```python
from build123d import *

# Parameters (mm, degrees)
CROQUIS1_R              = 25
SALIENTE_EXTRUIR1_DEPTH = 30


with BuildPart() as part:
    # Croquis1 → Saliente-Extruir1 (new body)
    with BuildSketch(Plane(origin=(0, 0, 0), x_dir=(1, 0, 0), z_dir=(0, 1, 0))):
        with BuildLine():
            Line((-65.797376832, 25.36524745), (-63.002208753, 26.454758997))
            ThreePointArc((-63.002208753, 26.454758997), (-56.557387251, 8.427488435), (-51.143577362, -9.935759386))
            Line((-51.143577362, -9.935759386), (-27.717597065, -3.966713114))
            ThreePointArc((-27.717597065, -3.966713114), (27.133039517, 6.913621813), (-26.236106677, -9.780935868))
            Line((-26.236106677, -9.780935868), (-49.662086973, -15.74998214))
            ThreePointArc((-49.662086973, -15.74998214), (-45.628225194, -34.464847013), (-42.660438023, -53.378081728))
            Line((-42.660438023, -53.378081728), (-45.636154363, -53.759017766))
            ThreePointArc((-45.636154363, -53.759017766), (-53.297041908, -13.580328562), (-65.797376832, 25.36524745))
        make_face()
        Circle(CROQUIS1_R, mode=Mode.SUBTRACT)
    extrude(amount=SALIENTE_EXTRUIR1_DEPTH)


solid = part.part
```
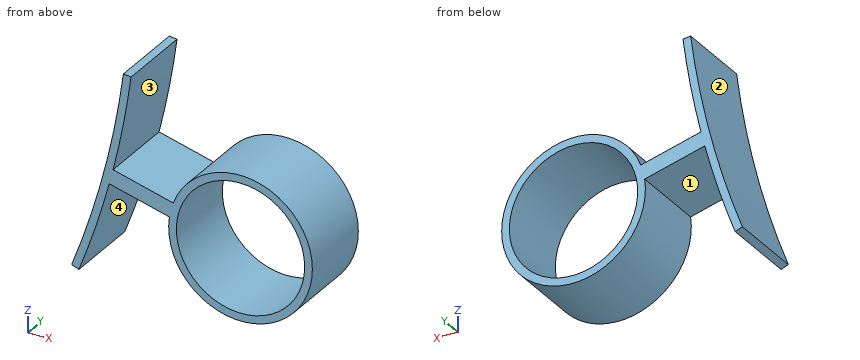
Geometry: final body of the model. Coordinates: model frame, mm. Face numbers are marked on the shaded views. A direction names the side the tool comes from. Round coordinates to 2 decimals unless told otherwise and drop trailing zeros. Order: outer loops, then holes, each group sorted by start corner. A loop starts at its lowest first (then second) coordinate and runs counter-clockwise, first axis right, second up. Notation, with made-up numbers: M 33,-1.75 L 77,-1.75 A7 cw 77,6.25 Z; hole C 59,-4.75 d11. An arc over 180 degrees is marked long. Use one line per item in the form item = value. Start each with the question number.
Q1. Mould query, pull axis X, two halves, no side actions, for the marked faces 1 and 2. Classes: +X half, -X half, draft (parallel to the pull), parting line (faces both ways), or undercut.
Q2. Cut plane C-C (y = 16.5). Return loops of the section in (x, z), and give its area (3 significant figures).
Q3. Cut plane A-A (x = 0). Return loops of the section in (y, z), and give its area (3 significant figures).
Q4. Pin query (flat end, axial travel): pin 1 Ø10 at (y, z) = (10.5, -6.5) entering from -X; pin 2 Ø5 at (y, z) = (24, 32.5) entering from +X; pin 3 Ø4 at (y, z) = (25.5, 42) entering from -X. Return the tip coordinate at first contact, or that it passes through.
Q5. Access query for the marked faces 3 and 4. Directions: +Z, -Z, +X, -X, +Y, -Y. A direction counts if a zero-diameter tool reaches every point of the face in a straight line with its end or side. Return the directions, or none.
Q6. Cut plane D-D (x = -13). Return loops of the section in (y, z).
Q7. Cut plane B-B (z = 18). Return loops of the section in (x, y), and give its area (3 significant figures).
Q8. Material intervals for line 1 (X direction, y = 19, z = 0); line 2 (X direction, y = 26.5, z = -19); line 3 (Z direction, x = 0, y = 13), sorted ascending. Write a range as [from, to].
Geometry results:
q1.face_1 = undercut
q1.face_2 = -X half
q2.outline = M -65.8,-25.37 L -63,-26.45 A338 ccw -51.14,9.94 L -27.72,3.97 A28 ccw long -26.24,9.78 L -49.66,15.75 A338 ccw -42.66,53.38 L -45.64,53.76 A335 cw Z; hole C 0,0 d50
q2.area = 891 mm^2
q3.outline = M 0,-28 L 30,-28 L 30,-25 L 0,-25 Z; M 0,25 L 30,25 L 30,28 L 0,28 Z
q3.area = 180 mm^2
q4.pin_1 = -60.74
q4.pin_2 = -45.53
q4.pin_3 = -47.69
q5.face_3 = +Y, -Y
q5.face_4 = -Z, +Y, -Y
q6.outline = M 0,-24.8 L 30,-24.8 L 30,-21.35 L 0,-21.35 Z; M 0,21.35 L 30,21.35 L 30,24.8 L 0,24.8 Z
q7.outline = M -52.2,0 L -49.12,0 L -49.12,30 L -52.2,30 Z; M -21.45,0 L -17.35,0 L -17.35,30 L -21.45,30 Z; M 17.35,0 L 21.45,0 L 21.45,30 L 17.35,30 Z
q7.area = 338 mm^2
q8.line_1 = [-57.06, -53.93], [-28, -25], [25, 28]
q8.line_2 = [-63.39, -60.2], [-20.57, -16.25], [16.25, 20.57]
q8.line_3 = [-28, -25], [25, 28]
